The model under review builds one solid part; all positions refer to its coordinate system, in mm. A direction names the side the tool comes from. Coordinates: 2 decimals unless noted, no trailing zeros. Loops run counter-clockwise (first coordinate to the right, second up) from the corner with the lowest first, then second, coordinate; pieces in that order, holes last. Notation, with made-up numbers: (51.25, 1.5) - (56.25, 1.5) arc R17 ccw to (56.25, 5.5) - close; hole circle Ø8 at (63, 33). An arc over 180 degrees is marked (long way). Use a Markdown table: item, result. Add a question column.
1) To check wall thickness, follow L1, parallel to X at y = -16.5, z = 8; L2, parallel to X at y = 21.5, z = 5.5; L3, parallel to Y at x = 186.5, z = 12.25. State the ranges of each line that lie inside material, in increasing order. Write a range as [from, to].
2) Add section A-A, the plane y = 26.5. Give the boundary of the cut face in (x, z).
3) Add section B-B, the plane x = -139. Give the boundary of the cut face in (y, z), and give its area (3 significant figures).
4) For faces 1 (the flat face through (155, 28, 8)), 2 (the flat face through (135, 28, 8)), 3 (the cylindrical face through (178.3, -24.8, 8.1)), 4 (the cylindrical face through (157.281, -37.594, 8.112)), 5 (the flat face through (-175, 20, 8)), list the 3-axis set-ups (+Z, -Z, +X, -X, +Y, -Y) from which the entire face can be reached by the end or side of a thin tool; tool diameter is ignored.
5) Add section C-C, the plane x = 30. Give the boundary of the cut face in (y, z), and give its area (3 significant figures).
6) The part is to be moulded in two halves that separate along Z. For faces 6 (the conical face through (-174.453, -8.362, 8.172)), 7 (the cylindrical face through (152.594, -22.281, 8.112)), 8 (the flat face through (-3, -1, 0)), say which applies: pulls with the +Z half, pulls with the -Z half, needs draft (parallel to the pull), parting line crosses it, or undercut.
7) Clearance check with flat-ended pins moving along their axes: pin 1 (4 mm diameter, centred on x = -64, z = 8, fed in from +Y); pin 2 (3 mm diameter, centred on x = -16.5, z = 13, fed in from -Y); pin 3 (2.5 mm diameter, centred on x = -186.5, y = 11.25, fed in from +Z); pin 4 (5 mm diameter, centred on y = 26, z = 6.5, fed in from +X). State where each tip first meets the part, or that it passes through.
```python
from build123d import *

# Parameters (mm, degrees)
F0_W     = 40
F0_H     = 20
F1_DEPTH = 16
F2_W     = 20
F2_H     = 16
F3_DEPTH = 16
F5_D     = 6.6
F5_DEPTH = 30
F5_TIP   = 1.9828400428
F6_R     = 8
F8_D     = 3.3
F8_DEPTH = 20
F8_TIP   = 0.9914200214
F10_D    = 3.3


with BuildPart() as f1:
    # F0 (on Top) → F1 (new body)
    with BuildSketch(Plane.XY):
        Polygon((195, -20), (195, 20), (-195, 20), (-195, -20), (-155, -20), (155, -20), align=None)
        with Locations((-175, -30)):
            Rectangle(F0_W, F0_H)
        with Locations((175, -30)):
            Rectangle(F0_W, F0_H)
    extrude(amount=F1_DEPTH)

    # F2 (on face) → F3 (join, through all)
    with BuildSketch(Plane.XY.offset(16)):
        with Locations((145, 28)):
            Rectangle(F2_W, F2_H)
        with Locations((0, 28)):
            Rectangle(F2_W, F2_H)
        with Locations((-145, 28)):
            Rectangle(F2_W, F2_H)
    extrude(amount=-F3_DEPTH)

    # F5
    with Locations(Plane.XZ.offset(40)):
        with Locations((-175, 8), (175, 8)):
            Hole(F5_D / 2, depth=F5_DEPTH)
            with Locations((0, 0, -(F5_DEPTH + F5_TIP / 2))):  # 118° drill point
                Cone(0, F5_D / 2, F5_TIP, mode=Mode.SUBTRACT)

    # F6
    f6_edges = [f1.edges().sort_by_distance(p)[0] for p in [
        (-155, -40, 8),
        (-155, -20, 8),
        (-195, -40, 8),
        (195, -40, 8),
        (155, -40, 8),
        (155, -20, 8),
    ]]
    fillet(f6_edges, radius=F6_R)

    # F8
    with Locations(Plane(origin=(0, 20, 0), x_dir=(-1, 0, 0), z_dir=(0, 1, 0))):
        with Locations((95, 8), (-95, 8)):
            Hole(F8_D / 2, depth=F8_DEPTH)
            with Locations((0, 0, -(F8_DEPTH + F8_TIP / 2))):  # 118° drill point
                Cone(0, F8_D / 2, F8_TIP, mode=Mode.SUBTRACT)

    # F10 (through all)
    with Locations(Plane.XY.offset(16)):
        with Locations((-186.5, 11.25), (-186.5, -31.25), (186.5, 11.25), (186.5, -31.25)):
            Hole(F10_D / 2)


solid = f1.part
```
From the geometry:
| question | item | result |
|---|---|---|
| 1 | L1 | x = [-195, -178.3], [-171.7, 171.7], [178.3, 195] |
| 1 | L2 | x = [-155, -135], [-10, 10], [135, 155] |
| 1 | L3 | y = [-40, -32.9], [-29.6, 9.6], [12.9, 20] |
| 2 | outline | (-155, 0) - (-135, 0) - (-135, 16) - (-155, 16) - close; (-10, 0) - (10, 0) - (10, 16) - (-10, 16) - close; (135, 0) - (155, 0) - (155, 16) - (135, 16) - close |
| 3 | outline | (-20, 0) - (36, 0) - (36, 16) - (-20, 16) - close |
| 3 | area | 896 mm^2 |
| 4 | face 1 | +Z, -Z, +X, +Y |
| 4 | face 2 | +Z, -Z, +Y |
| 4 | face 3 | -Y |
| 4 | face 4 | +Z, -Z, -Y |
| 4 | face 5 | +Z, -Z, -X, +Y |
| 5 | outline | (-20, 0) - (20, 0) - (20, 16) - (-20, 16) - close |
| 5 | area | 640 mm^2 |
| 6 | face 6 | undercut |
| 6 | face 7 | needs draft |
| 6 | face 8 | pulls with the -Z half |
| 7 | pin 1 | stops at y = 20 |
| 7 | pin 2 | stops at y = -20 |
| 7 | pin 3 | passes through |
| 7 | pin 4 | stops at x = 155 |
